from build123d import *

# Parameters (mm, degrees)
EXTRUDE_1_DEPTH     = 1
EXTRUDE_2_DEPTH     = 4
CUT_EXTRUDE_1_DEPTH = 9


with BuildPart() as part:
    # Sketch 1 → Extrude 1 (new body)
    with BuildSketch(Plane(origin=(0, 0, 0), x_dir=(1, 0, 0), z_dir=(0, 1, 0))):
        Polygon((-2, -2), (-1, 2), (-3, 2), (-3, -2), align=None)
        Polygon((1, 2), (-1, 2), (-2, -2), (2, -2), align=None)
        Polygon((3, 2), (1, 2), (2, -2), (3, -2), align=None)
    extrude(amount=EXTRUDE_1_DEPTH)

    # Sketch 1_3 → Extrude 2 (add)
    with BuildSketch(Plane(origin=(0, 0, 0), x_dir=(1, 0, 0), z_dir=(0, 1, 0))):
        Polygon((-2, -2), (-1, 2), (-3, 2), (-3, -2), align=None)
        Polygon((3, 2), (1, 2), (2, -2), (3, -2), align=None)
    extrude(amount=EXTRUDE_2_DEPTH)

    # Sketch 2 → Cut-Extrude 1 (cut)
    with BuildSketch(Plane(origin=(3, 0, 0), x_dir=(0, 0, -1), z_dir=(1, 0, 0))):
        Polygon((2, 4), (-2, 1), (-2, 4), align=None)
    extrude(amount=-CUT_EXTRUDE_1_DEPTH, mode=Mode.SUBTRACT)


solid = part.part
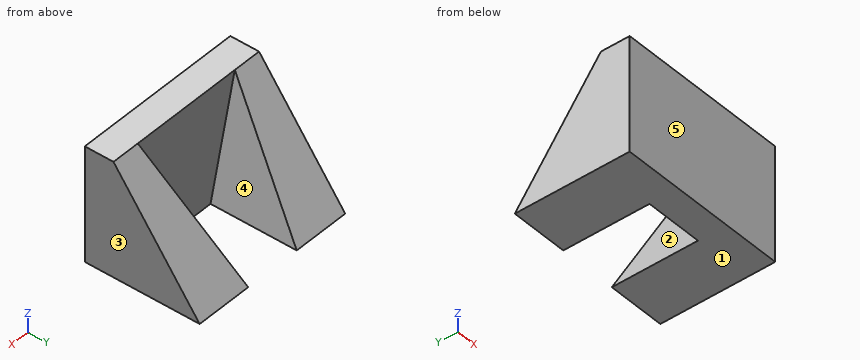
For this review, take the finished solid that the model builds, in its own axes (mm). Face numbers are marked on the shaded views. A direction names the side the tool comes from. Round coordinates to 2 decimals unless told otherwise and drop trailing zeros. Loops run counter-clockwise (first coordinate to the right, second up) from the corner with the lowest first, then second, coordinate; pieces in that order, holes last. Notation, with made-up numbers: (51.25, 87.5) - (95.25, 87.5) arc R28 cw to (95.25, 124.5) - close; hole circle Ø8 at (-39.75, -29.5). An arc over 180 degrees is marked (long way). Use one line per item in the form item = value.
1) We need section D-D on x = -1.45. Write out the cut boundary in (y, z).
Solutions:
outline = (0, -2) - (4, -2) - (2.65, -0.2) - (1, -0.2) - (1, 2) - (0, 2) - close
2) We need section A-A on y = 1.3. Write out the cut boundary in (x, z), then the cut area to 3 significant figures.
Solutions:
outline = (-3, -2) - (-1, -2) - (-1.9, 1.6) - (-3, 1.6) - close; (1, -2) - (3, -2) - (3, 1.6) - (1.9, 1.6) - close
area = 11.2 mm2
3) Tool access review of the marked faces 4 and 5: name each direction out of +Z, -Z, +X, -X, +Y, -Y from which nothing blocks a thin tool from reaching the whole face with its end or side.
Solutions:
face_4 = +Z, +Y
face_5 = +Z, -Z, +X, -X, -Y
4) Wall thickness on probe 1 along Y at (x, z) = (-0.55, 1.65); probe 2 along X at (y, z) = (1.8, 0.2); probe 3 along X at (y, z) = (2.9, -1.1) (3 decimals): over which ranges is each line inside the solid? List them lowest first.
Solutions:
probe_1 = 0 to 1
probe_2 = -3 to -1.55, 1.55 to 3
probe_3 = -3 to -1.225, 1.225 to 3
5) We need section B-B on z = 1.2. Write out the cut boundary in (x, y).
Solutions:
outline = (-3, 0) - (3, 0) - (3, 1.6) - (1.8, 1.6) - (1.8, 1) - (-1.8, 1) - (-1.8, 1.6) - (-3, 1.6) - close
6) We need section C-C on y = 2.65. Write out the cut boundary in (x, z), then the cut area to 3 significant figures.
Solutions:
outline = (-3, -2) - (-1, -2) - (-1.45, -0.2) - (-3, -0.2) - close; (1, -2) - (3, -2) - (3, -0.2) - (1.45, -0.2) - close
area = 6.39 mm2
7) Mouldability with a two-part tool opening along X and no side actions: class the marked faces 1, 2 and 3 as pulls with the +X half, pulls with the -X half, needs draft (parallel to the pull), parting line crosses it, or undercut.
Solutions:
face_1 = needs draft
face_2 = undercut
face_3 = pulls with the +X half
